The listing builds one solid part. Answer for the finished solid, in the listing's coordinates (mm). A direction names the side the tool comes from. Round coordinates to 2 decimals unless told otherwise and drop trailing zeros. Write each loop counter-clockwise with the first axis right and the second up, starting at its lowest first coordinate (ties: lowest second). Pieces come first, ordered by that corner, then holes.
(1) A cutting plane is placed at C-C, the plane x = 69.5. Give the vertices of the cut face in (y, z).
(2) Find the intervals of material crossed by probe 1 along X at (y, z) = (6.5, 2); probe 2 along Z at (x, y) = (31, 9); probe 3 along Y at (x, z) = (7.5, -1), in increasing order.
(3) Each of these flat-tipped pins is pushed along its axis until it touches: pin 1 Ø1.5 at (y, z) = (-1, 0.5) entering from -X; pin 2 Ø5 at (x, y) = (56.5, 11) entering from -Z. Where does it stop, or does it pass through?
(4) For faces 1 (the face through (45.891, 6.696, 0.021)), 2 (the face through (48, -7, 1.5)), 3 (the face through (48, -7, -1.5)), determine the directions among +Z, -Z, +X, -X, +Y, -Y from which every point of the face is accessible in a straight line to the end or side of a thin tool.
(5) A cutting plane is placed at B-B, the plane y = 7. Give the vertices of the cut face in (x, z).
(6) A cutting plane is placed at A-A, the plane z = -0.25. Give the vertices of the cut face in (x, y).
from build123d import *

# Parameters (mm, degrees)
F0_W     = 35
F0_H     = 10
F1_DEPTH = 3
F3_DEPTH = 1.5


with BuildPart() as f1:
    # F0 (on Right) → F1 (new body)
    with BuildSketch(Plane.YZ):
        Rectangle(F0_W, F0_H)
    extrude(amount=F1_DEPTH)

    # F2 (on Top) → F3 (join, symmetric)
    with BuildSketch(Plane.XY):
        Polygon((3, -10.985037), (3, -14), (93, -5), (93, 5), (3, 14), (3, 10.985037), (90, 2.285037), (90, -2.285037), align=None)
    extrude(amount=F3_DEPTH, both=True)


solid = f1.part
Solutions:
1. outline: (-7.35, -1.5) - (-4.34, -1.5) - (-4.34, 1.5) - (-7.35, 1.5) - close; (4.34, -1.5) - (7.35, -1.5) - (7.35, 1.5) - (4.34, 1.5) - close
2. probe 1: x = 0 to 3
2. probe 2: z = -1.5 to 1.5
2. probe 3: y = -13.55 to -10.54, 10.54 to 13.55
3. pin 1: stops at x = 0
3. pin 2: stops at z = -1.5
4. face 1: +Z, -Z
4. face 2: +Z, +X, +Y, -Y
4. face 3: -Z, +X, +Y, -Y
5. outline: (0, -5) - (3, -5) - (3, 5) - (0, 5) - close; (42.85, -1.5) - (73, -1.5) - (73, 1.5) - (42.85, 1.5) - close
6. outline: (0, -17.5) - (3, -17.5) - (3, -14) - (93, -5) - (93, 5) - (3, 14) - (3, 17.5) - (0, 17.5) - close; hole (3, -10.99) - (90, -2.29) - (90, 2.29) - (3, 10.99) - close
